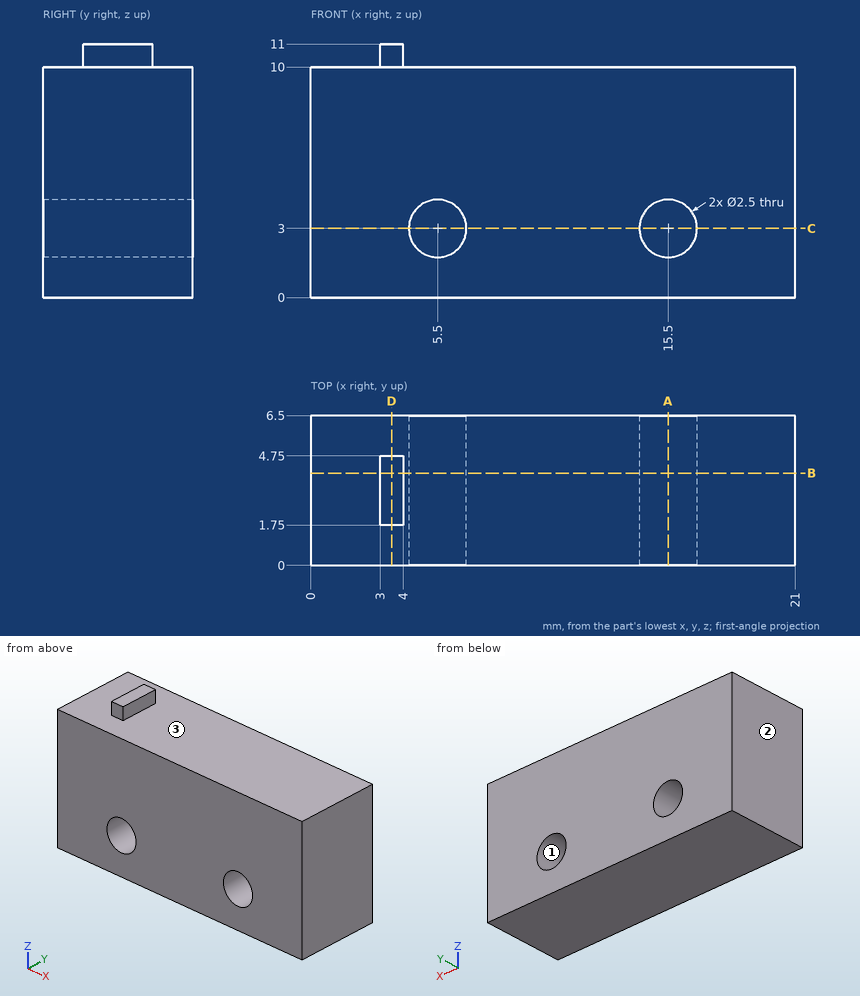
Geometry: see drawing. Coordinates: mm, zero at the bounding-box minimum. Coordinates: 2 decimals unless noted, no trailing zeros. Loops run counter-clockwise (first coordinate to the right, second up) from the corner with the lowest first, then second, coordinate; pieces in that order, holes last. Notation, with made-up numbers: (22, 30) - (33, 30) arc R7 ccw to (33, 36) - close; hole circle Ø5 at (54.25, 10.5). An arc over 180 degrees is marked (long way). Put each result on its own line as item: value. Start each with the question number.
Q1. Cut plane C-C, the plane z = 3. Return loops of the section in (x, y).
Q2. Line query: line 1 (X direction, y = 3, z = 3.5); line 2 (Z direction, x = 5.5, y = 3); line 3 (X direction, y = 1.5, z = 2.75). Output: solid intervals per line, ascending.
Q3. Pin query (flat end, axial travel): pin 1 Ø0.8 at (y, z) = (3.5, 10.5) entering from +X; pin 2 Ø0.5 at (x, z) = (3.5, 10.5) entering from -Y; pin 3 Ø0.5 at (x, z) = (3.5, 10.5) entering from +Y; pin 4 Ø3 at (x, z) = (15.5, 3) entering from -Y. Return the tip coordinate at first contact, or that it passes through.
Q4. Cut plane B-B, the plane y = 4. Return loops of the section in (x, z), and give its area (3 significant figures).
Q5. Pull-direction query (X, two-part tool) for the marked faces 1, 2 and 3; classes: released by +X, released by -X, zero draft, split by the parting line, or undercut.
Q6. Cut plane A-A, the plane x = 15.5. Return loops of the section in (y, z), and give its area (4 significant figures).
Q7. Cut plane D-D, the plane x = 3.5. Return loops of the section in (y, z).
Filled sheet:
1. outline: (0, 0) - (4.25, 0) - (4.25, 6.5) - (0, 6.5) - close; (6.75, 0) - (14.25, 0) - (14.25, 6.5) - (6.75, 6.5) - close; (16.75, 0) - (21, 0) - (21, 6.5) - (16.75, 6.5) - close
2. line 1: 0 to 4.35, 6.65 to 14.35, 16.65 to 21
2. line 2: 0 to 1.75, 4.25 to 10
2. line 3: 0 to 4.28, 6.72 to 14.28, 16.72 to 21
3. pin 1: x = 4
3. pin 2: y = 1.75
3. pin 3: y = 4.75
3. pin 4: y = 0
4. outline: (0, 0) - (21, 0) - (21, 10) - (4, 10) - (4, 11) - (3, 11) - (3, 10) - (0, 10) - close; hole circle Ø2.5 at (5.5, 3); hole circle Ø2.5 at (15.5, 3)
4. area: 201 mm²
5. face 1: undercut
5. face 2: released by -X
5. face 3: zero draft
6. outline: (0, 0) - (6.5, 0) - (6.5, 1.75) - (0, 1.75) - close; (0, 4.25) - (6.5, 4.25) - (6.5, 10) - (0, 10) - close
6. area: 48.75 mm²
7. outline: (0, 0) - (6.5, 0) - (6.5, 10) - (4.75, 10) - (4.75, 11) - (1.75, 11) - (1.75, 10) - (0, 10) - close
